```python
from build123d import *

# Parameters (mm, degrees)
PAD_DEPTH     = 20
SKETCH001_R   = 1.6
SKETCH001_W   = 8.873669
SKETCH001_H   = 5
SKETCH001_W_2 = 10.362093
POCKET_DEPTH  = 5
FILLET_R      = 4


with BuildPart() as part:
    # Sketch → Pad (new body)
    with BuildSketch(Plane.XZ):
        Polygon((0, 11.366025), (23.382686, -2.133975), (22.882686, -3), (2, 9.056624), (2, 0), (-6, 0), (-6, 2), (0, 2), align=None)
    extrude(amount=PAD_DEPTH)

    # Sketch001 (on Face7 of Pad) → Pocket (cut)
    with BuildSketch(Plane(origin=(0, 0, 2), x_dir=(-1, 0, 0), z_dir=(0, 0, 1))):
        with Locations((3, 10)):
            Circle(SKETCH001_R)
        with Locations((4.436834, 2.5)):
            Rectangle(SKETCH001_W, SKETCH001_H)
        with Locations((5.181046, 17.5)):
            Rectangle(SKETCH001_W_2, SKETCH001_H)
    extrude(amount=-POCKET_DEPTH, mode=Mode.SUBTRACT)

    # Fillet
    fillet_edges = [part.edges().sort_by_distance(p)[0] for p in [
        (-6, -5, 1),
        (-6, -15, 1),
    ]]
    fillet(fillet_edges, radius=FILLET_R)


solid = part.part
```
Source: CAD feature listing. Evaluate the final solid. Frame: model axes, mm. A direction names the side the tool comes from. Round coordinates to 2 decimals unless told otherwise and drop trailing zeros. Order: outer loops, then holes, each group sorted by start corner. A loop starts at its lowest first (then second) coordinate and runs counter-clockwise, first axis right, second up. Notation, with made-up numbers: (25, 53.25) -> (40, 53.25) arc R28 ccw to (40, 90.25) -> close; hole circle Ø10 at (78, 89.5). An arc over 180 degrees is marked (long way). Use CSV: the item, a comma, the result in double quotes.
(1) Access query for faces 4 (the face through (-1.7, -8.8, 2)), 5 (the face through (0, -2, 1)), 6 (the face through (-1, -10, 0)), 7 (the face through (-1, -15, 1)), 8 (the face through (2, -10, 5)). Directions: +Z, -Z, +X, -X, +Y, -Y. A direction counts if a zero-diameter tool reaches every point of the face in a straight line with its end or side. Return the directions, or none.
Report:
face 4,"+Z, -X, +Y, -Y"
face 5,"+Z, -Z, -X, +Y"
face 6,"-Z, -X, +Y, -Y"
face 7,"+Z, -Z, -X, -Y"
face 8,"-Z, +Y, -Y"
(2) First-contact query: pin 1 Ø1 at (y, z) = (-7.5, 0) entering from +X; pin 2 Ø8 at (y, z) = (-17.5, 0) entering from -X; pin 3 Ø5 at (y, z) = (-12, 5.5) entering from -X; pin 4 Ø2 at (x, z) = (10, 1.5) entering from +Y. Flat tips, straight axial feed; report the tip coordinate or a pass-through.
Report:
pin 1,"x = 20.55"
pin 2,"x = -5.12"
pin 3,"x = 0"
pin 4,"through"
(3) Ray query, L1, parallel to X at y = -10, z = 1.35; L2, parallel to X at y = -10, z = 1.5; L3, parallel to Y at x = -3, z = 1.2. Return the intervals inside material, ascending.
Report:
L1,"-6 to -4.6, -1.4 to 2, 15.35 to 17.35"
L2,"-6 to -4.6, -1.4 to 2, 15.09 to 17.09"
L3,"-14.87 to -11.6, -8.4 to -5.13"
(4) Section A-A on y = -10. Return the cut outline in (x, z).
Report:
outline,"(-6, 0) -> (-4.6, 0) -> (-4.6, 2) -> (-6, 2) -> close; (-1.4, 0) -> (2, 0) -> (2, 9.06) -> (22.88, -3) -> (23.38, -2.13) -> (0, 11.37) -> (0, 2) -> (-1.4, 2) -> close"
(5) Pull-direction query (Y, two-part tool) for faces 1 (the face through (-4.797, -13.859, 0.986)), 2 (the face through (-2.65, -8.44, 1.01)), 3 (the face through (11.53, -9.86, 4.71)); classes: +Y half, -Y half, draft (parallel to the pull), parting line (faces both ways), or undercut.
Report:
face 1,"-Y half"
face 2,"undercut"
face 3,"draft"
(6) Section D-D on z = 6.75. Return the cut outline in (x, y).
Report:
outline,"(0, -20) -> (2, -20) -> (2, 0) -> (0, 0) -> close; (6, -20) -> (8, -20) -> (8, 0) -> (6, 0) -> close"
(7) Section C-C on y = -4. Return the cut outline in (x, z).
Report:
outline,"(0, 0) -> (2, 0) -> (2, 9.06) -> (22.88, -3) -> (23.38, -2.13) -> (0, 11.37) -> close"
(8) Section B-B on x = -3. Return the cut outline in (y, z), and give its area (3 significant figures).
Report:
outline,"(-14.87, 0) -> (-11.6, 0) -> (-11.6, 2) -> (-14.87, 2) -> close; (-8.4, 0) -> (-5.13, 0) -> (-5.13, 2) -> (-8.4, 2) -> close"
area,"13.1 mm^2"
